from build123d import *

# Parameters (mm, degrees)
SKETCH1_W                       = 63.5
SKETCH1_H                       = 24.13
BOSS_EXTRUDE1_DEPTH             = 4.064
BOSS_EXTRUDE2_REACH             = 14.065
BOSS_EXTRUDE2_DIRECTION_2_REACH = 14.065
SKETCH4_R                       = 8.636
CUT_EXTRUDE1_DEPTH              = 4.064
CUT_EXTRUDE1_DEPTH_BACK         = 5.064
FILLET1_R                       = 2.54
CUT_EXTRUDE2_DEPTH              = 25.1300001
BOSS_EXTRUDE3_DEPTH             = 2.54
BOSS_EXTRUDE4_DEPTH             = 2.54
BOSS_EXTRUDE5_DEPTH             = 3.81
CUT_EXTRUDE3_DEPTH              = 8.8740001
BOSS_EXTRUDE6_START             = -23.114
SKETCH12_W                      = 44.831
SKETCH12_H                      = 27.027043781
BOSS_EXTRUDE6_DEPTH             = 23.114
BOSS_EXTRUDE7_DEPTH             = 7.874
CUT_EXTRUDE4_START              = -6.219751
CUT_EXTRUDE4_DEPTH              = 6.219751
CUT_EXTRUDE5_DEPTH              = 27.027044
SKETCH17_W                      = 6.9977
SKETCH17_H                      = 3.556
BOSS_EXTRUDE8_DEPTH             = 13.97
SKETCH18_W                      = 6.389869694
SKETCH18_H                      = 3.556
BOSS_EXTRUDE9_DEPTH             = 13.97
SKETCH19_W                      = 31.75
SKETCH19_H                      = 7.112
CUT_EXTRUDE6_DEPTH              = 13.97
CUT_EXTRUDE7_REACH              = 52.797
SKETCH20_R                      = 1.7145
FILLET2_R                       = 2.54
FILLET3_R                       = 2.54
FILLET4_R                       = 2.54
SKETCH21_W                      = 12
SKETCH21_H                      = 11
SKETCH21_W_2                    = 11
SKETCH21_H_2                    = 12
BOSS_EXTRUDE10_DEPTH            = 3.7
BOSS_EXTRUDE11_DEPTH            = 11
FILLET5_R                       = 2.54
SKETCH23_R                      = 2.325
CUT_EXTRUDE8_DEPTH              = 4.7000001


with BuildPart() as part:
    # Sketch1 → Boss-Extrude1 (new body)
    with BuildSketch(Plane(origin=(0, 0, 0), x_dir=(1, 0, 0), z_dir=(0, 1, 0))):
        Rectangle(SKETCH1_W, SKETCH1_H)
    extrude(amount=BOSS_EXTRUDE1_DEPTH)

    # Boss-Extrude2: up to this face of the body (flat: up to its plane)
    boss_extrude2_end = Plane(part.part.faces().sort_by_distance((0, 2.032, 12.065))[0])
    # Sketch2 → Boss-Extrude2 (add, up to the picked face)
    with BuildSketch(Plane.XY, mode=Mode.PRIVATE) as boss_extrude2_sk1:
        with BuildLine():
            Line((0, 4.064), (-26.716755185, 4.064))
            Line((-26.716755185, 4.064), (-31.571041118, 27.367716778))
            ThreePointArc((-31.571041118, 27.367716778), (-27.221246487, 47.076161415), (-11.87173913, 60.180974548))
            ThreePointArc((-11.87173913, 60.180974548), (-8.566242036, 58.774955714), (-9.97226087, 55.46945862))
            ThreePointArc((-9.97226087, 55.46945862), (-26.181898149, 25.654914521), (0, 4.064))
        make_face()
    boss_extrude2_tool1 = split(extrude(boss_extrude2_sk1.sketch, amount=BOSS_EXTRUDE2_REACH, mode=Mode.PRIVATE), bisect_by=boss_extrude2_end, keep=Keep.BOTH, mode=Mode.PRIVATE)
    add(boss_extrude2_tool1.solids().sort_by_distance((-9.165723, 58.533271, 0))[0])

    # Boss-Extrude2 direction 2: up to this face of the body (flat: up to its plane)
    boss_extrude2_direction_2_end = Plane(part.part.faces().sort_by_distance((0, 2.032, -12.065))[0])
    # Sketch2 → Boss-Extrude2 direction 2 (add, up to the picked face)
    with BuildSketch(Plane.XY, mode=Mode.PRIVATE) as boss_extrude2_direction_2_sk1:
        with BuildLine():
            Line((0, 4.064), (-26.716755185, 4.064))
            Line((-26.716755185, 4.064), (-31.571041118, 27.367716778))
            ThreePointArc((-31.571041118, 27.367716778), (-27.221246487, 47.076161415), (-11.87173913, 60.180974548))
            ThreePointArc((-11.87173913, 60.180974548), (-8.566242036, 58.774955714), (-9.97226087, 55.46945862))
            ThreePointArc((-9.97226087, 55.46945862), (-26.181898149, 25.654914521), (0, 4.064))
        make_face()
    boss_extrude2_direction_2_tool1 = split(extrude(boss_extrude2_direction_2_sk1.sketch, amount=-BOSS_EXTRUDE2_DIRECTION_2_REACH, mode=Mode.PRIVATE), bisect_by=boss_extrude2_direction_2_end, keep=Keep.BOTH, mode=Mode.PRIVATE)
    add(boss_extrude2_direction_2_tool1.solids().sort_by_distance((-9.165723, 58.533271, 0))[0])

    # Sketch4 → Cut-Extrude1 (cut, two sides)
    with BuildSketch(Plane(origin=(0, 4.064, 0), x_dir=(1, 0, 0), z_dir=(0, 1, 0))) as cut_extrude1_sk:
        Circle(SKETCH4_R)
    extrude(amount=CUT_EXTRUDE1_DEPTH, mode=Mode.SUBTRACT)
    extrude(cut_extrude1_sk.sketch, amount=-CUT_EXTRUDE1_DEPTH_BACK, mode=Mode.SUBTRACT)

    # Fillet1
    fillet1_edges = [part.edges().sort_by_distance(p)[0] for p in [
        (-8.636, 5.50091846, 0),
        (6.106574162, 4.064, 6.106574162),
    ]]
    fillet(fillet1_edges, radius=FILLET1_R)

    # Sketch6 → Cut-Extrude2 (cut, through all)
    with BuildSketch(Plane.XY.offset(12.065)):
        Polygon((-31.75, 4.064), (-26.716755185, 4.064), (-25.870202757, 0), (-31.75, 0), align=None)
    extrude(amount=-CUT_EXTRUDE2_DEPTH, mode=Mode.SUBTRACT)

    # Sketch8 → Boss-Extrude3 (add)
    with BuildSketch(Plane.XY.offset(12.065)):
        with BuildLine():
            Line((31.75, 0), (31.75, 7.874))
            Line((31.75, 7.874), (-4.274632474, 7.874))
            ThreePointArc((-4.274632474, 7.874), (-23.508790492, 29.710248048), (-9.97226087, 55.46945862))
            ThreePointArc((-9.97226087, 55.46945862), (-8.566242036, 58.774955714), (-11.87173913, 60.180974548))
            ThreePointArc((-11.87173913, 60.180974548), (-27.221246487, 47.076161415), (-31.571041118, 27.367716778))
            Line((-31.571041118, 27.367716778), (-25.870202757, 0))
            Line((-25.870202757, 0), (31.75, 0))
        make_face()
    extrude(amount=BOSS_EXTRUDE3_DEPTH)

    # Sketch9 → Boss-Extrude4 (add)
    with BuildSketch(Plane(origin=(0, 0, -12.065), x_dir=(-1, 0, 0), z_dir=(0, 0, -1))):
        with BuildLine():
            Line((-31.75, 0), (-31.75, 7.874))
            Line((-31.75, 7.874), (4.274632474, 7.874))
            ThreePointArc((4.274632474, 7.874), (23.508790492, 29.710248048), (9.97226087, 55.46945862))
            ThreePointArc((9.97226087, 55.46945862), (8.566242036, 58.774955714), (11.87173913, 60.180974548))
            ThreePointArc((11.87173913, 60.180974548), (27.221246487, 47.076161415), (31.571041118, 27.367716778))
            Line((31.571041118, 27.367716778), (25.870202757, 0))
            Line((25.870202757, 0), (-31.75, 0))
        make_face()
    extrude(amount=BOSS_EXTRUDE4_DEPTH)

    # Sketch10 → Boss-Extrude5 (add)
    with BuildSketch(Plane(origin=(0, 4.064, 0), x_dir=(1, 0, 0), z_dir=(0, 1, 0))):
        with BuildLine():
            Line((10.218295125, 14.605), (10.218295125, 12.065))
            ThreePointArc((10.218295125, 12.065), (22.283295125, 0), (10.218295125, -12.065))
            Line((10.218295125, -12.065), (10.218295125, -14.605))
            ThreePointArc((10.218295125, -14.605), (24.823295125, 0), (10.218295125, 14.605))
        make_face()
    extrude(amount=BOSS_EXTRUDE5_DEPTH)

    # Sketch11 → Cut-Extrude3 (cut, through all)
    with BuildSketch(Plane(origin=(0, 7.874, 0), x_dir=(1, 0, 0), z_dir=(0, 1, 0))):
        with BuildLine():
            Line((10.218295125, 14.605), (31.75, 14.605))
            Line((31.75, 14.605), (31.75, -14.605))
            Line((31.75, -14.605), (10.218295125, -14.605))
            ThreePointArc((10.218295125, -14.605), (24.823295125, 0), (10.218295125, 14.605))
        make_face()
    extrude(amount=-CUT_EXTRUDE3_DEPTH, mode=Mode.SUBTRACT)

    # Sketch12 → Boss-Extrude6 (add)
    with BuildSketch(Plane.XZ.offset(BOSS_EXTRUDE6_START)):
        with Locations((-8.8011, -28.11852189)):
            Rectangle(SKETCH12_W, SKETCH12_H)
    extrude(amount=BOSS_EXTRUDE6_DEPTH)

    # Sketch13 → Boss-Extrude7 (add)
    with BuildSketch(Plane.XZ):
        Polygon((10.218295125, -14.605), (13.6144, -14.605), (13.6144, -13.335525526), align=None)
    extrude(amount=-BOSS_EXTRUDE7_DEPTH)

    # Sketch14 → Cut-Extrude4 (cut)
    with BuildSketch(Plane.XY.offset(-14.605).offset(CUT_EXTRUDE4_START)):
        with BuildLine():
            Line((0, 13.017313502), (18.620278687, 13.017313502))
            Line((18.620278687, 13.017313502), (17.716686498, 30.734))
            ThreePointArc((17.716686498, 30.734), (-12.527589163, 43.261589163), (0, 13.017313502))
        make_face()
    extrude(amount=CUT_EXTRUDE4_DEPTH, mode=Mode.SUBTRACT)

    # Sketch16 → Cut-Extrude5 (cut)
    with BuildSketch(Plane.XY.offset(-14.605)):
        Polygon((-31.2166, 23.114), (-30.684969694, 23.114), (-25.870202757, 0), (-31.2166, 0), align=None)
    extrude(amount=-CUT_EXTRUDE5_DEPTH, mode=Mode.SUBTRACT)

    # Sketch17 → Boss-Extrude8 (add)
    with BuildSketch(Plane(origin=(0, 23.114, 0), x_dir=(1, 0, 0), z_dir=(0, 1, 0))):
        with Locations((10.11555, 34.413750632)):
            Rectangle(SKETCH17_W, SKETCH17_H)
    extrude(amount=BOSS_EXTRUDE8_DEPTH)

    # Sketch18 → Boss-Extrude9 (add)
    with BuildSketch(Plane(origin=(0, 23.114, 0), x_dir=(1, 0, 0), z_dir=(0, 1, 0))):
        with Locations((-27.490034847, 34.413750632)):
            Rectangle(SKETCH18_W, SKETCH18_H)
    extrude(amount=BOSS_EXTRUDE9_DEPTH)

    # Sketch19 → Cut-Extrude6 (cut)
    with BuildSketch(Plane(origin=(0, 37.084, 0), x_dir=(1, 0, 0), z_dir=(0, 1, 0))):
        with Locations((-8.8392, 36.191750632)):
            Rectangle(SKETCH19_W, SKETCH19_H)
    extrude(amount=-CUT_EXTRUDE6_DEPTH, mode=Mode.SUBTRACT)

    # Sketch20 → Cut-Extrude7 (cut, up to next)
    with BuildSketch(Plane(origin=(0, 0, -36.191750632), x_dir=(-1, 0, 0), z_dir=(0, 0, -1)), mode=Mode.PRIVATE) as cut_extrude7_sk1:
        with Locations((27.75585, 30.734)):
            Circle(SKETCH20_R)
    cut_extrude7_tool1 = extrude(cut_extrude7_sk1.sketch, amount=-CUT_EXTRUDE7_REACH, mode=Mode.PRIVATE) & part.part
    add(cut_extrude7_tool1.solids().sort_by_distance((-27.75585, 30.734, -36.191751))[0], mode=Mode.SUBTRACT)
    # Sketch20 → Cut-Extrude7 (cut, up to next)
    with BuildSketch(Plane(origin=(0, 0, -36.191750632), x_dir=(-1, 0, 0), z_dir=(0, 0, -1)), mode=Mode.PRIVATE) as cut_extrude7_sk2:
        with Locations((-10.11555, 30.734)):
            Circle(SKETCH20_R)
    cut_extrude7_tool2 = extrude(cut_extrude7_sk2.sketch, amount=-CUT_EXTRUDE7_REACH, mode=Mode.PRIVATE) & part.part
    add(cut_extrude7_tool2.solids().sort_by_distance((10.11555, 30.734, -36.191751))[0], mode=Mode.SUBTRACT)

    # Fillet2
    fillet2_edges = [part.edges().sort_by_distance(p)[0] for p in [
        (10.3251, 23.114, -36.191750632),
    ]]
    fillet(fillet2_edges, radius=FILLET2_R)

    # Fillet3
    fillet3_edges = [part.edges().sort_by_distance(p)[0] for p in [
        (-27.699584847, 23.114, -36.191750632),
    ]]
    fillet(fillet3_edges, radius=FILLET3_R)

    # Fillet4
    fillet4_edges = [part.edges().sort_by_distance(p)[0] for p in [
        (13.6144, 37.084, -34.413750632),
        (-30.684969694, 37.084, -34.413750632),
    ]]
    fillet(fillet4_edges, radius=FILLET4_R)

    # Sketch21 → Boss-Extrude10 (add)
    with BuildSketch(Plane.XZ):
        with Locations((-19.870202757, 20.105)):
            Rectangle(SKETCH21_W, SKETCH21_H)
        with Locations((4.218295125, 20.105)):
            Rectangle(SKETCH21_W, SKETCH21_H)
        with Locations((19.1144, -27.812319928)):
            Rectangle(SKETCH21_W_2, SKETCH21_H_2)
    extrude(amount=-BOSS_EXTRUDE10_DEPTH)

    # Sketch22 → Boss-Extrude11 (add)
    with BuildSketch(Plane.XY.offset(14.605)):
        Polygon((-25.870202757, 3.7), (-26.640932084, 3.7), (-25.870202757, 0), align=None)
    extrude(amount=BOSS_EXTRUDE11_DEPTH)

    # Fillet5
    fillet5_edges = [part.edges().sort_by_distance(p)[0] for p in [
        (10.218295125, 1.85, 14.605),
        (-13.870202757, 1.85, 25.605),
        (-13.870202757, 1.85, 14.605),
        (10.218295125, 1.85, 25.605),
        (-1.781704875, 1.85, 14.605),
        (-1.781704875, 1.85, 25.605),
        (13.6144, 1.85, -33.812319928),
        (13.6144, 1.85, -21.812319928),
        (24.6144, 1.85, -21.812319928),
        (24.6144, 1.85, -33.812319928),
        (-26.25556742, 1.85, 25.605),
    ]]
    fillet(fillet5_edges, radius=FILLET5_R)

    # Sketch23 → Cut-Extrude8 (cut, through all)
    with BuildSketch(Plane(origin=(0, 3.7, 0), x_dir=(1, 0, 0), z_dir=(0, 1, 0))):
        with Locations((20.0034, 27.812319928)):
            Circle(SKETCH23_R)
        with Locations((-20.228306672, -20.994)):
            Circle(SKETCH23_R)
        with Locations((4.218295125, -20.994)):
            Circle(SKETCH23_R)
    extrude(amount=-CUT_EXTRUDE8_DEPTH, mode=Mode.SUBTRACT)


solid = part.part
Can you work these out from the model? Positions are in its coordinate system, mm. A direction names the side the tool comes from. Give positions to 0.01 mm unless a question says otherwise; leave off trailing zeros. Order: outer loops, then holes, each group sorted by start corner. A loop starts at its lowest first (then second) coordinate and runs counter-clockwise, first axis right, second up. Notation, with made-up numbers: M 40.5,-2 L 71.5,-2 A26 ccw 71.5,33 Z; hole C 71.25,33 d8. An arc over 180 degrees is marked long. Use one line per item in the form item = value. Start each with the question number.
Item 1: If we section it at C-C (y = 15.5): Write out the boundary of the cut face in (x, z) (3 decimals).
Item 2: We'd pull the mould along Y, two halves only. Please class faces 1 (the flat face through (-18.9, 3.7, 18.8)), 2 (the cylindrical face through (8.48, 31.25, -34.44)), 3 (the cylindrical face through (23.851, 1.876, -22.537)): +Y half, -Y half, draft (parallel to the pull), parting line (faces both ways), or undercut.
Item 3: For faces 4 (the cylindrical face through (-29.34, 30.08, -34.44)), 5 (the flat face through (-1.782, 2, 20)), 6 (the cylindrical face through (22.28, 5.94, -0.27)), 7 (the cylindrical face through (-8.628, 1.067, -0.38)), 8 (the cylindrical face through (14.38, 1.88, -21.09)), which set-ups out of +Z, -Z, +X, -X, +Y, -Y let a thin tool reach every point of the face, with its end or its side?
Item 4: If we section it at B-B (x = 5.5): State how many separate pieces and enclosed holes the cut face has, then the cut area to 3 significant figures.
Item 5: If we section it at A-A (z = 20): Write out the boundary of the cut face in (x, y).
Item 6: If I drill on line 1 along Z through (x, y) = (-25.5, 31.5) (3 decimals); line 2 along Z through (x, y) = (8, 33); line 3 along Y through (x, z) = (3, 10.5), over which ranges is the centre line in solid material (lowest first)?
Item 7: Will these pins go through, and if not, where does the flat tip stop? pin 1 Ø1.8 at (x, y) = (18.5, 1.5) entering from -Z; pin 2 Ø8 at (y, z) = (11.5, -18.5) entering from -X; pin 3 Ø9 at (x, z) = (17.5, -30) entering from +Y; pin 4 Ø5 at (x, z) = (-1.5, -5.5) entering from -Y.
Outcome:
q1.outline = M -29.099,-41.632 L 13.614,-41.632 L 13.614,-20.825 L -9.045,-20.825 L -9.045,-14.605 L -17.017,-14.605 L -17.017,-12.065 L -21.891,-12.065 L -21.891,12.065 L -17.017,12.065 L -17.017,14.605 L -29.099,14.605 Z
q2.face_1 = +Y half
q2.face_2 = undercut
q2.face_3 = draft
q3.face_4 = -Z
q3.face_5 = +Z, +Y, -Y
q3.face_6 = +Y
q3.face_7 = -Y
q3.face_8 = +X, +Y, -Y
q4.separate_pieces = 3
q4.enclosed_holes = 0
q4.area = 669 mm2
q5.outline = M -26.64,3.7 L -25.87,0 L -22.33,0 L -22.33,3.7 Z; M -18.13,0 L -13.87,0 L -13.87,3.7 L -18.13,3.7 Z; M -1.78,0 L 2.12,0 L 2.12,3.7 L -1.78,3.7 Z; M 6.32,0 L 10.22,0 L 10.22,3.7 L 6.32,3.7 Z
q6.line_1 = -36.192 to -32.636, -14.605 to -12.065, 12.065 to 14.605
q6.line_2 = -36.19 to -32.64
q6.line_3 = 0 to 4.05
q7.pin_1 = -33.81
q7.pin_2 = -29.1
q7.pin_3 = 23.11
q7.pin_4 = through
